from build123d import *

# Parameters (mm, degrees)
EXTRUDE_1_DEPTH     = 50
SKETCH_1_3_R        = 30
CUT_EXTRUDE_1_DEPTH = 40


with BuildPart() as part:
    # Sketch 1 → Extrude 1 (new body)
    with BuildSketch(Plane.XY):
        with BuildLine():
            Line((0, -40), (-250, -40))
            ThreePointArc((-250, -40), (-290, 0), (-250, 40))
            Line((-250, 40), (0, 40))
            ThreePointArc((0, 40), (40, 0), (0, -40))
        make_face()
    extrude(amount=EXTRUDE_1_DEPTH)

    # Sketch 1_3 → Cut-Extrude 1 (cut)
    with BuildSketch(Plane.XY):
        with Locations((-250, 0)):
            Circle(SKETCH_1_3_R)
        Circle(SKETCH_1_3_R)
        with Locations((-187.5, 0)):
            Circle(SKETCH_1_3_R)
        with Locations((-62.5, 0)):
            Circle(SKETCH_1_3_R)
        with Locations((-125, 0)):
            Circle(SKETCH_1_3_R)
    extrude(amount=CUT_EXTRUDE_1_DEPTH, mode=Mode.SUBTRACT)


solid = part.part
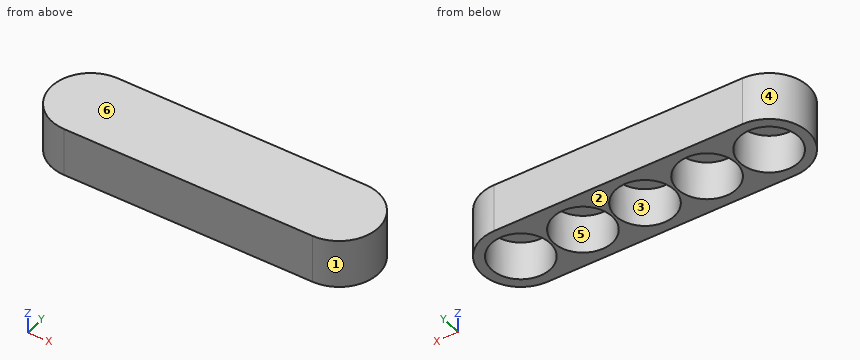
Model file for the job. Use its own axes, mm. Face numbers are marked on the shaded views. A direction names the side the tool comes from. Round coordinates to 2 decimals unless told otherwise and drop trailing zeros. Loops run counter-clockwise (first coordinate to the right, second up) from the corner with the lowest first, then second, coordinate; pieces in that order, holes last.
1. Drop flat-ended pins along their axis: P1, Ø6, axis at y = -7.5, z = 42, coming from the -X side; P2, Ø18, axis at x = -183, y = -1.5, coming from the -Z side; P3, Ø5, axis at y = -31, z = 10, coming from the -X side. Give the stop position or say it passes through.
Check values:
P1: stops at x = -289.75
P2: stops at z = 40
P3: stops at x = -278.07
2. Band-saw the part on A-A, the plane z = 10. List the corners of the cut face in (x, y), and give its area (3 significant figures).
Check values:
outline: (-250, -40) - (0, -40) arc R40 ccw to (0, 40) - (-250, 40) arc R40 ccw to start; hole circle Ø60 at (-250, 0); hole circle Ø60 at (-187.5, 0); hole circle Ø60 at (-125, 0); hole circle Ø60 at (-62.5, 0); hole circle Ø60 at (0, 0)
area: 10,900 mm2
3. Tool access for the marked faces 5 and 6: list every direction of +Z, -Z, +X, -X, +Y, -Y with a clear straight run to the whole face (end or side of a thin tool).
Check values:
face 5: -Z
face 6: +Z, +X, -X, +Y, -Y
4. Band-saw the part on B-B, the plane x = -232. List the corners of the cut face in (y, z).
Check values:
outline: (-40, 0) - (-24, 0) - (-24, 40) - (24, 40) - (24, 0) - (40, 0) - (40, 50) - (-40, 50) - close
5. Band-saw the part on C-C, the plane y = 0. List the corners of the cut face in (x, z).
Check values:
outline: (-290, 0) - (-280, 0) - (-280, 40) - (-220, 40) - (-220, 0) - (-217.5, 0) - (-217.5, 40) - (-157.5, 40) - (-157.5, 0) - (-155, 0) - (-155, 40) - (-95, 40) - (-95, 0) - (-92.5, 0) - (-92.5, 40) - (-32.5, 40) - (-32.5, 0) - (-30, 0) - (-30, 40) - (30, 40) - (30, 0) - (40, 0) - (40, 50) - (-290, 50) - close
6. Band-saw the part on D-D, the plane z = 44.5. List the corners of the cut face in (x, y), and give its area (3 significant figures).
Check values:
outline: (-250, -40) - (0, -40) arc R40 ccw to (0, 40) - (-250, 40) arc R40 ccw to start
area: 25,000 mm2
7. Mould opens along X. For the marked faces 1, 2, 3 and 4 say: +X half, -X half, draft (parallel to the pull), parting line (faces both ways), or undercut.
Check values:
face 1: +X half
face 2: draft
face 3: undercut
face 4: -X half
8. Wall check: probe 1 along X at (y, z) = (-1, 28); probe 2 along Y at (x, z) = (-187.5, 25.5); probe 3 along X at (y, z) = (-23, 5). Give the ranges that are in metal, low to high.
Check values:
probe 1: x = -289.99 to -279.98, -220.02 to -217.48, -157.52 to -154.98, -95.02 to -92.48, -32.52 to -29.98, 29.98 to 39.99
probe 2: y = -40 to -30, 30 to 40
probe 3: x = -282.73 to -269.26, -230.74 to -206.76, -168.24 to -144.26, -105.74 to -81.76, -43.24 to -19.26, 19.26 to 32.73
